CAD build for the part. Positions are in the model's coordinates, mm. Give positions to 0.01 mm unless a question says otherwise; leave off trailing zeros. Loops run counter-clockwise (first coordinate to the right, second up) from the corner with the lowest first, then second, coordinate; pieces in that order, holes last.
Item 1: Mould opens along X. For faces 1 (the cylindrical face through (3.728, -5.847, 82.602)), 2 (the flat face through (-0.335, 8.72, 5.227)), 3 (the cylindrical face through (-1.389, -10.577, 82.58)) say: released by +X, released by -X, zero draft, split by the parting line, or undercut.
Item 2: Saw through at B-B on z = 13.5. Give the cut face in (x, y).
Item 3: Saw through at A-A on y = 0. Give the cut face in (x, z), plus the area to 3 significant figures.
Item 4: Probe probe 1 along X at (y, z) = (0, 125); probe 2 along Z at (x, y) = (7.25, 1.25). List the from-to ranges inside material, lowest first.
Item 5: Drop flat-ended pins along their axis: P1, Ø6, axis at y = 5.5, z = 83, coming from the +X side; P2, Ø5, axis at y = 8.5, z = 132.5, coming from the +X side; P3, Ø10, axis at y = 6.5, z = 146, coming from the -X side; P4, Ø8.5, axis at x = 0, y = 0, coming from the +Z side. Give the stop position or say it passes through.
Autodesk Inventor part; units mm, degrees
ref_plane "Start Plane" through (0, 0, -4.4541) normal (0, 0, 1) x (1, 0, 0)
ref_plane "End Plane" through (0, 0, 172.086) normal (0, 0, 1) x (1, 0, 0)
ref_plane "Work Plane4" through (-9.2, -5.4006, 178.0712) normal (0.6032, 0.3541, 0.7147) x (0.7878, -0.1245, -0.6032)
ref_plane "Start Plane" through (0, 0, -4.4541) normal (0, 0, 1) x (1, 0, 0)
ref_plane "End Plane" through (0, 0, 172.086) normal (0, 0, 1) x (1, 0, 0)
sketch "Sketch" plane through (0, 0, 0) normal (0, 0, 1) x (1, 0, 0)
  circle A0 centre (0, 0) radius 6.9342
  circle A1 centre (0, 0) radius 10.668
  dimension "d0" = 21.336
  dimension "d1" = 3.7338
extrude "Body" add sketch "Sketch" along normal up to surface (176.5401 mm away) from surface at -4.4541
sketch "Sketch3" plane through (0, 0, 0) normal (0, 0, 1) x (1, 0, 0)
  line L0 (0, 0) -> (10, 0)
ref_plane "Work Plane3" through (0, 0, 0) normal (0, -1, 0) x (1, 0, 0)
sketch "Sketch4" plane through (0, 0, 0) normal (0, -1, 0) x (1, 0, 0)
  line L0 (-2, -4.4541) -> (12, -4.4541)
  line L1 (-2, 172.086) -> (12, 172.086)
  dimension "d7" = 176.5401
ref_plane "Work Plane4" through (-9.2, -5.4006, 178.0712) normal (0.6032, 0.3541, 0.7147) x (0.7878, -0.1245, -0.6032)
split "Split1" plane through (-9.2, -5.4006, 178.0712) removes the side toward (0.6032, 0.3541, 0.7147)
ref_plane "Work Plane5" through (10.1246, -3.3615, 178.7912) normal (-0.686, 0.2278, 0.691) x (0.7217, 0.0924, 0.686)
split "Split2" plane through (10.1246, -3.3615, 178.7912) removes the side toward (-0.686, 0.2278, 0.691)
ref_plane "Work Plane6" through (-3.2893, -10.1482, 174.4387) normal (0.1659, 0.5117, 0.843) x (0.9851, -0.046, -0.1659)
split "Split3" plane through (-3.2893, -10.1482, 174.4387) removes the side toward (0.1659, 0.5117, 0.843)
ref_plane "Work Plane7" through (-9.2, -5.4006, -10.4394) normal (0.6032, 0.3541, -0.7147) x (-0.2753, -0.7486, -0.6032)
split "Split4" plane through (-9.2, -5.4006, -10.4394) removes the side toward (0.6032, 0.3541, -0.7147)
ref_plane "Work Plane8" through (10.1246, -3.3615, -11.1594) normal (-0.686, 0.2278, -0.691) x (-0.5231, 0.5057, 0.686)
split "Split5" plane through (10.1246, -3.3615, -11.1594) removes the side toward (-0.686, 0.2278, -0.691)
ref_plane "Work Plane9" through (-3.2893, -10.1482, -6.8069) normal (0.1659, 0.5117, -0.843) x (0.8248, -0.5406, -0.1659)
split "Split6" plane through (-3.2893, -10.1482, -6.8069) removes the side toward (0.1659, 0.5117, -0.843)
equation "\"d0\" = G_H"
equation "\"d1\" = G_T"
equation "\"d2\" = G_L"
equation "\"G_H\" = 21.336"
equation "\"G_T\" = 3.7338"
equation "\"G_L\" = 176.5401"
equation "\"G_OFFSET_START\" = 4.45413"
equation "\"G_OFFSET_END\" = 4.45413"
equation "\"d4\" = -G_OFFSET_START"
equation "\"d5\" = G_OFFSET_END + B_L"
equation "\"B_L\" = 167.63184"
properties part number "ANSI - 1/2 x 0.147 - 6.95" material "Steel, Mild"
Results below:
1. face 1: undercut
1. face 2: released by +X
1. face 3: split by the parting line
2. outline: circle Ø21.34 at (0, 0); hole circle Ø13.87 at (0, 0)
3. outline: (-10.67, 10.59) - (-6.93, 6.88) - (-6.93, 160.75) - (-10.67, 157.04) - close; (6.93, 5.85) - (10.67, 9) - (10.67, 158.63) - (6.93, 161.78) - close
3. area: 1,130 mm2
4. probe 1: x = -10.67 to -6.93, 6.93 to 10.67
4. probe 2: z = 6.74 to 160.89
5. P1: stops at x = 10.37
5. P2: stops at x = 8.82
5. P3: stops at x = -10.56
5. P4: passes through
